Read the model definition and answer for the solid it produces. Units are mm, in the model's axes. A direction names the side the tool comes from. Coordinates: 2 decimals unless noted, no trailing zeros. Loops run counter-clockwise (first coordinate to the right, second up) from the corner with the lowest first, then second, coordinate; pieces in that order, holes last.
from build123d import *

# Parameters (mm, degrees)
BOSS_EXTRUDE1_DEPTH                               = 31.75
CBORE_FOR_5_16_SOCKET_HEAD_CAP_SCREW1_D           = 8.2042
CBORE_FOR_5_16_SOCKET_HEAD_CAP_SCREW1_CBORE_D     = 12.7
CBORE_FOR_5_16_SOCKET_HEAD_CAP_SCREW1_CBORE_DEPTH = 9.525
F_3_8_0_375_CLEARANCE_DOWEL_HOLE2_D               = 9.525
SKETCH9_W                                         = 23.721553131
SKETCH9_H                                         = 31.75
CUT_EXTRUDE1_DEPTH                                = 1.27


with BuildPart() as part:
    # Sketch1 → Boss-Extrude1 (new body)
    with BuildSketch(Plane.XY):
        with BuildLine():
            Line((0, 0), (12.7, 0))
            ThreePointArc((12.7, 0), (37.719, -25.019), (62.738, 0))
            Line((62.738, 0), (91.313, 0))
            Line((91.313, 0), (91.313, -31.496))
            Line((91.313, -31.496), (0, -31.496))
            Line((0, -31.496), (0, 0))
        make_face()
    extrude(amount=BOSS_EXTRUDE1_DEPTH)

    # CBORE for 5/16 Socket Head Cap Screw1 (through all)
    with Locations(Plane(origin=(0, -31.496, 0), x_dir=(-1, 0, 0), z_dir=(0, -1, 0))):
        with Locations((-7.1247, -15.875), (-81.788, -15.875)):
            CounterBoreHole(CBORE_FOR_5_16_SOCKET_HEAD_CAP_SCREW1_D / 2, CBORE_FOR_5_16_SOCKET_HEAD_CAP_SCREW1_CBORE_D / 2, CBORE_FOR_5_16_SOCKET_HEAD_CAP_SCREW1_CBORE_DEPTH)

    # 3/8 (0.375) Clearance Dowel Hole2 (through all)
    with Locations(Plane(origin=(0, -31.496, 0), x_dir=(-1, 0, 0), z_dir=(0, -1, 0))):
        with Locations((-69.088, -15.875)):
            Hole(F_3_8_0_375_CLEARANCE_DOWEL_HOLE2_D / 2)

    # Sketch9 → Cut-Extrude1 (cut)
    with BuildSketch(Plane(origin=(0, 0, 0), x_dir=(1, 0, 0), z_dir=(0, 1, 0))):
        with Locations((11.860776566, -15.875)):
            Rectangle(SKETCH9_W, SKETCH9_H)
    extrude(amount=-CUT_EXTRUDE1_DEPTH, mode=Mode.SUBTRACT)

    # Chamfer1
    # the kernel refuses this chamfer: 2.54 mm, written as the material it takes off along each edge
    with BuildSketch(Plane(origin=(89.619666667, -29.802666667, 30.056666667), x_dir=(0, -0.7071067811865476, -0.7071067811865476), z_dir=(0.5773502691896247, -0.5773502691896263, 0.5773502691896263)), Plane(origin=(1.693333333, -29.802666667, 1.693333333), x_dir=(0.7071067811865474, 0, -0.7071067811865477), z_dir=(-0.5773502691896264, -0.5773502691896247, -0.5773502691896262))) as chamfer1_piece_1:
        Polygon((-1.796051224, -1.036950658), (1.796051224, -1.036950658), (0, 2.073901316), align=None)
    extrude(amount=3.226233304, mode=Mode.SUBTRACT)
    with BuildSketch(Plane(origin=(89.619666667, -29.802666667, 1.693333333), x_dir=(0, -0.7071067811865474, 0.7071067811865477), z_dir=(0.5773502691896246, -0.5773502691896264, -0.5773502691896262)), Plane(origin=(1.693333333, -29.802666667, 30.056666667), x_dir=(0.7071067811865476, 0, 0.7071067811865476), z_dir=(-0.5773502691896263, -0.5773502691896247, 0.5773502691896263))) as chamfer1_piece_2:
        Polygon((-1.796051224, 1.036950658), (1.796051224, 1.036950658), (0, -2.073901316), align=None)
    extrude(amount=3.226233304, mode=Mode.SUBTRACT)
    with BuildSketch(Plane(origin=(91.313, 6.532074789, 31.75), x_dir=(-0.9996219169112968, 0, 0.02749587661058591), z_dir=(0, -1, 0))) as chamfer1_piece_3:
        with BuildLine():
            Line((2.612829916, 0), (-0.143629773, 2.608879196))
            Line((-0.143629773, 2.608879196), (-0.194410567, 2.607482405))
            ThreePointArc((-0.194410567, 2.607482405), (-0.086688237, 1.304030487), (-0.050780793, -0.001396791))
            Line((-0.050780793, -0.001396791), (0.001396791, -0.050780793))
            ThreePointArc((0.001396791, -0.050780793), (1.306824068, -0.01487335), (2.614226706, -0.050780793))
            Line((2.614226706, -0.050780793), (2.612829916, 0))
        make_face()
    extrude(amount=44.560149579, mode=Mode.SUBTRACT)
    with BuildSketch(Plane(origin=(91.313, -31.496, -6.532074789), x_dir=(-0.9996219169112968, -0.02749587661058591, 0), z_dir=(0, 0, 1)), Plane(origin=(0, -31.496, -6.532074789), x_dir=(-0.027495876610586358, 0.9996219169112968, 0), z_dir=(0, 0, 1))) as chamfer1_piece_4:
        with BuildLine():
            Line((2.612829916, 0), (-0.143629773, -2.608879196))
            Line((-0.143629773, -2.608879196), (-0.194410567, -2.607482405))
            ThreePointArc((-0.194410567, -2.607482405), (-0.086688237, -1.304030487), (-0.050780793, 0.001396791))
            Line((-0.050780793, 0.001396791), (0.001396791, 0.050780793))
            ThreePointArc((0.001396791, 0.050780793), (1.306824068, 0.01487335), (2.614226706, 0.050780793))
            Line((2.614226706, 0.050780793), (2.612829916, 0))
        make_face()
    extrude(amount=44.814149579, mode=Mode.SUBTRACT)
    with BuildSketch(Plane(origin=(0, -38.028074789, 0), x_dir=(-0.027495876610586365, 0, 0.9996219169112968), z_dir=(0, 1, 0))) as chamfer1_piece_5:
        with BuildLine():
            Line((2.612829916, 0), (-0.143629773, 2.608879196))
            Line((-0.143629773, 2.608879196), (-0.194410567, 2.607482405))
            ThreePointArc((-0.194410567, 2.607482405), (-0.086688237, 1.304030487), (-0.050780793, -0.001396791))
            Line((-0.050780793, -0.001396791), (0.001396791, -0.050780793))
            ThreePointArc((0.001396791, -0.050780793), (1.306824068, -0.01487335), (2.614226706, -0.050780793))
            Line((2.614226706, -0.050780793), (2.612829916, 0))
        make_face()
    extrude(amount=43.290149579, mode=Mode.SUBTRACT)
    with BuildSketch(Plane(origin=(0, -38.028074789, 31.75), x_dir=(-0.0274958766105864, 0, -0.9996219169112968), z_dir=(0, 1, 0))) as chamfer1_piece_6:
        with BuildLine():
            Line((2.612829916, 0), (-0.143629773, -2.608879196))
            Line((-0.143629773, -2.608879196), (-0.194410567, -2.607482405))
            ThreePointArc((-0.194410567, -2.607482405), (-0.086688237, -1.304030487), (-0.050780793, 0.001396791))
            Line((-0.050780793, 0.001396791), (0.001396791, 0.050780793))
            ThreePointArc((0.001396791, 0.050780793), (1.306824068, 0.01487335), (2.614226706, 0.050780793))
            Line((2.614226706, 0.050780793), (2.612829916, 0))
        make_face()
    extrude(amount=43.290149579, mode=Mode.SUBTRACT)
    with BuildSketch(Plane(origin=(97.845074789, -31.496, 31.75), x_dir=(0, 0.9996219169112966, 0.027495876610585942), z_dir=(-1, 0, 0))) as chamfer1_piece_7:
        with BuildLine():
            Line((2.612829916, 0), (-0.143629773, 2.608879196))
            Line((-0.143629773, 2.608879196), (-0.194410567, 2.607482405))
            ThreePointArc((-0.194410567, 2.607482405), (-0.086688237, 1.304030487), (-0.050780793, -0.001396791))
            Line((-0.050780793, -0.001396791), (0.001396791, -0.050780793))
            ThreePointArc((0.001396791, -0.050780793), (1.306824068, -0.01487335), (2.614226706, -0.050780793))
            Line((2.614226706, -0.050780793), (2.612829916, 0))
        make_face()
    extrude(amount=104.377149579, mode=Mode.SUBTRACT)
    with BuildSketch(Plane(origin=(91.313, 6.532074789, 0), x_dir=(-0.9996219169112968, 0, -0.027495876610586324), z_dir=(0, -1, 0))) as chamfer1_piece_8:
        with BuildLine():
            Line((2.612829916, 0), (-0.143629773, -2.608879196))
            Line((-0.143629773, -2.608879196), (-0.194410567, -2.607482405))
            ThreePointArc((-0.194410567, -2.607482405), (-0.086688237, -1.304030487), (-0.050780793, 0.001396791))
            Line((-0.050780793, 0.001396791), (0.001396791, 0.050780793))
            ThreePointArc((0.001396791, 0.050780793), (1.306824068, 0.01487335), (2.614226706, 0.050780793))
            Line((2.614226706, 0.050780793), (2.612829916, 0))
        make_face()
    extrude(amount=44.560149579, mode=Mode.SUBTRACT)
    with BuildSketch(Plane(origin=(97.845074789, -31.496, 0), x_dir=(0, 0.9996219169112966, -0.0274958766105864), z_dir=(-1, 0, 0))) as chamfer1_piece_9:
        with BuildLine():
            Line((2.612829916, 0), (-0.143629773, -2.608879196))
            Line((-0.143629773, -2.608879196), (-0.194410567, -2.607482405))
            ThreePointArc((-0.194410567, -2.607482405), (-0.086688237, -1.304030487), (-0.050780793, 0.001396791))
            Line((-0.050780793, 0.001396791), (0.001396791, 0.050780793))
            ThreePointArc((0.001396791, 0.050780793), (1.306824068, 0.01487335), (2.614226706, 0.050780793))
            Line((2.614226706, 0.050780793), (2.612829916, 0))
        make_face()
    extrude(amount=104.377149579, mode=Mode.SUBTRACT)


solid = part.part
Q1. A cutting plane is placed at C-C (z = 13). Give the vertices of the cut face in (x, y).
Findings below:
outline: (0, -28.96) - (1.46, -30.42) - (1.46, -21.97) - (4.2, -21.97) - (4.2, -1.27) - (0, -1.27) - close; (10.05, -21.97) - (12.79, -21.97) - (12.79, -31.5) - (65.29, -31.5) - (65.29, 0) - (62.74, 0) arc R25.02 cw to (12.73, -1.27) - (10.05, -1.27) - close; (72.88, -31.5) - (76.13, -31.5) - (76.13, -21.97) - (78.86, -21.97) - (78.86, 0) - (72.88, 0) - close; (84.71, -21.97) - (87.45, -21.97) - (87.45, -31.5) - (88.77, -31.5) - (91.31, -28.96) - (91.31, 0) - (84.71, 0) - close
Q2. A cutting plane is placed at A-A (y = -18). Count the separate pieces of the cut face and the enclosed holes in it, then the cut area to 3 significant figures.
Findings below:
separate pieces: 2
enclosed holes: 3
area: 1,610 mm2
Q3. A cutting plane is placed at D-D (x = 71.5). Give the vertices of the cut face in (y, z).
Findings below:
outline: (-31.5, 2.54) - (-28.96, 0) - (0, 0) - (0, 11.77) - (-31.5, 11.77) - close; (-31.5, 19.98) - (0, 19.98) - (0, 31.75) - (-28.96, 31.75) - (-31.5, 29.21) - close
Q4. A cutting plane is placed at B-B (z = 4.5). Give the vertices of the cut face in (x, y), then the cut area to 3 significant figures.
Findings below:
outline: (0, -28.96) - (2.54, -31.5) - (88.77, -31.5) - (91.31, -28.96) - (91.31, 0) - (62.74, 0) arc R25.02 cw to (12.73, -1.27) - (0, -1.27) - close
area: 1,870 mm2
Q5. Which of the six approach directions +Z, -Z, +X, -X, +Y, -Y give full straight-line access (tool end or side, diameter ignored) to faces 1 (the face through (89.779, -29.705, 29.995)), 2 (the face through (5, -1.27, 12)), 3 (the face through (3, -21.971, 17))?
Findings below:
face 1: +Z, +X, -Y
face 2: +Z, -Z, -X, +Y
face 3: -Y
Q6. Determine the mould class of faces 4 (the face through (85.7, -10.83, 14.64)), 5 (the face through (0, -15, 16)), 6 (the face through (46.26, -30.208, 1.252)) for opening direction X: +X half, -X half, draft (parallel to the pull), parting line (faces both ways), or undercut.
Findings below:
face 4: undercut
face 5: -X half
face 6: draft
Q7. Flat-ended cylindrical pins translate along their axes: pin 1 Ø4 at (x, z) = (8.5, 18) entering from -Y; pin 2 Ø10.5 at (x, z) = (7.12, 15.88) entering from +Y; pin 3 Ø2 at (x, z) = (21.5, 28.5) entering from +Y; pin 4 Ø7.5 at (x, z) = (7.12, 15.88) entering from -Y. Find the tip coordinate at first contact, or state that the pin passes through.
Findings below:
pin 1: stops at y = -21.97
pin 2: stops at y = -1.27
pin 3: stops at y = -18.15
pin 4: passes through
Q8. Straight lines are drawn through the part: probe 1 along X at (y, z) = (-28, 17); probe 2 along X at (y, z) = (-22.5, 10); probe 3 along Z at (x, y) = (82, -26.5). For each, find the intervals that lie inside material, in ascending order.
Findings below:
probe 1: x = 0 to 0.88, 13.37 to 64.46, 73.72 to 75.54, 88.04 to 91.31
probe 2: x = 0 to 4.71, 9.53 to 26.78, 48.66 to 79.38, 84.2 to 91.31
probe 3: z = 0 to 9.53, 22.22 to 31.75
